```python
from build123d import *

# Parameters (mm, degrees)
SKETCH1_R           = 8
BOSS_EXTRUDE1_DEPTH = 40
CHAMFER1_SIZE       = 10
SKETCH2_R           = 8
BOSS_EXTRUDE2_DEPTH = 40
CUT_EXTRUDE2_REACH  = 134.076
SKETCH4_W           = 40
SKETCH4_H           = 10
FILLET4_R           = 10
CUT_EXTRUDE9_REACH  = 154.84
CUT_EXTRUDE10_REACH = 153.921
FILLET5_R           = 10
CUT_EXTRUDE11_REACH = 156.208
SKETCH15_R          = 12.5


with BuildPart() as part:
    # Sketch1 → Boss-Extrude1 (new body)
    with BuildSketch(Plane(origin=(0, 0, 0), x_dir=(1, 0, 0), z_dir=(0, 1, 0))):
        with BuildLine():
            Line((0, 0), (0, 144))
            Line((0, 144), (-6, 144))
            Line((-6, 144), (-6, 24))
            Line((-6, 24), (-26, 24))
            ThreePointArc((-26, 24), (-38, 12), (-26, 0))
            Line((-26, 0), (0, 0))
        make_face()
        with Locations(Location((-26, 12, 0), (0, 0, 270))):
            Circle(SKETCH1_R, mode=Mode.SUBTRACT)
    extrude(amount=BOSS_EXTRUDE1_DEPTH)

    # Chamfer1
    chamfer1_edges = [part.edges().sort_by_distance(p)[0] for p in [
        (-3, 40, -144),
        (-3, 0, -144),
    ]]
    chamfer(chamfer1_edges, length=CHAMFER1_SIZE)

    # Sketch2 → Boss-Extrude2 (add, through all)
    with BuildSketch(Plane(origin=(0, 40, 0), x_dir=(1, 0, 0), z_dir=(0, 1, 0))):
        with BuildLine():
            ThreePointArc((0, 0), (12, -12), (24, 0))
            Line((24, 0), (24, 24))
            Line((24, 24), (0, 24))
            Line((0, 24), (0, 0))
        make_face()
        with Locations(Location((12, 0, 0), (0, 0, 270))):
            Circle(SKETCH2_R, mode=Mode.SUBTRACT)
    extrude(amount=-BOSS_EXTRUDE2_DEPTH)

    # Sketch4 → Cut-Extrude2 (cut, up to next)
    with BuildSketch(Plane(origin=(0, 0, -24), x_dir=(-1, 0, 0), z_dir=(0, 0, -1)), mode=Mode.PRIVATE) as cut_extrude2_sk1:
        with Locations((26, 35)):
            Rectangle(SKETCH4_W, SKETCH4_H)
    cut_extrude2_tool1 = extrude(cut_extrude2_sk1.sketch, amount=-CUT_EXTRUDE2_REACH, mode=Mode.PRIVATE) & part.part
    # Sketch4 → Cut-Extrude2 (cut, up to next)
    with BuildSketch(Plane(origin=(0, 0, -24), x_dir=(-1, 0, 0), z_dir=(0, 0, -1)), mode=Mode.PRIVATE) as cut_extrude2_sk2:
        with Locations((26, 5)):
            Rectangle(SKETCH4_W, SKETCH4_H)
    cut_extrude2_tool2 = extrude(cut_extrude2_sk2.sketch, amount=-CUT_EXTRUDE2_REACH, mode=Mode.PRIVATE) & part.part
    # Sketch4 → Cut-Extrude2 (cut, up to next)
    with BuildSketch(Plane(origin=(0, 0, -24), x_dir=(-1, 0, 0), z_dir=(0, 0, -1)), mode=Mode.PRIVATE) as cut_extrude2_sk3:
        with Locations((-20, 5)):
            Rectangle(SKETCH4_W, SKETCH4_H)
    cut_extrude2_tool3 = extrude(cut_extrude2_sk3.sketch, amount=-CUT_EXTRUDE2_REACH, mode=Mode.PRIVATE) & part.part
    # Sketch4 → Cut-Extrude2 (cut, up to next)
    with BuildSketch(Plane(origin=(0, 0, -24), x_dir=(-1, 0, 0), z_dir=(0, 0, -1)), mode=Mode.PRIVATE) as cut_extrude2_sk4:
        with Locations((-20, 35)):
            Rectangle(SKETCH4_W, SKETCH4_H)
    cut_extrude2_tool4 = extrude(cut_extrude2_sk4.sketch, amount=-CUT_EXTRUDE2_REACH, mode=Mode.PRIVATE) & part.part
    add(cut_extrude2_tool1.solids().sort_by_distance((-26, 35, -24))[0], mode=Mode.SUBTRACT)
    add(cut_extrude2_tool2.solids().sort_by_distance((-26, 5, -24))[0], mode=Mode.SUBTRACT)
    add(cut_extrude2_tool3.solids().sort_by_distance((20, 5, -24))[0], mode=Mode.SUBTRACT)
    add(cut_extrude2_tool4.solids().sort_by_distance((20, 35, -24))[0], mode=Mode.SUBTRACT)

    # Fillet4
    fillet4_edges = [part.edges().sort_by_distance(p)[0] for p in [
        (-6, 20, -24),
    ]]
    fillet(fillet4_edges, radius=FILLET4_R)

    # Sketch13 → Cut-Extrude9 (cut, up to next)
    with BuildSketch(Plane.ZY.offset(6), mode=Mode.PRIVATE) as cut_extrude9_sk1:
        Polygon((0, 30), (-10, 40), (0, 40), align=None)
    cut_extrude9_tool1 = extrude(cut_extrude9_sk1.sketch, amount=-CUT_EXTRUDE9_REACH, mode=Mode.PRIVATE) & part.part
    # Sketch13 → Cut-Extrude9 (cut, up to next)
    with BuildSketch(Plane.ZY.offset(6), mode=Mode.PRIVATE) as cut_extrude9_sk2:
        Polygon((0, 10), (0, 0), (-10, 0), align=None)
    cut_extrude9_tool2 = extrude(cut_extrude9_sk2.sketch, amount=-CUT_EXTRUDE9_REACH, mode=Mode.PRIVATE) & part.part
    add(cut_extrude9_tool1.solids().sort_by_distance((-6, 36.666667, -3.333333))[0], mode=Mode.SUBTRACT)
    add(cut_extrude9_tool2.solids().sort_by_distance((-6, 3.333333, -3.333333))[0], mode=Mode.SUBTRACT)

    # Sketch14 → Cut-Extrude10 (cut, up to next)
    with BuildSketch(Plane(origin=(0, 30, 0), x_dir=(1, 0, 0), z_dir=(0, 1, 0)), mode=Mode.PRIVATE) as cut_extrude10_sk1:
        with BuildLine():
            Line((12, 12), (0, 12))
            Line((0, 12), (0, 24))
            Line((0, 24), (24, 24))
            Line((24, 24), (24, 0))
            ThreePointArc((24, 0), (20.485281374, 8.485281374), (12, 12))
        make_face()
    cut_extrude10_tool1 = extrude(cut_extrude10_sk1.sketch, amount=-CUT_EXTRUDE10_REACH, mode=Mode.PRIVATE) & part.part
    add(cut_extrude10_tool1.solids().sort_by_distance((12.903097, 30, -17.158841))[0], mode=Mode.SUBTRACT)

    # Fillet5
    # the kernel refuses this fillet: 10 mm, written as the material it adds along each edge
    with BuildSketch(Plane(origin=(0, 30, -12), x_dir=(0, 0, -1), z_dir=(0, -1, 0))) as fillet5_piece_1:
        with BuildLine():
            CenterArc((FILLET5_R, FILLET5_R), FILLET5_R, 180, 90)
            Line((0, FILLET5_R), (0, 0))
            Line((0, 0), (FILLET5_R, 0))
        make_face()
    extrude(amount=20)
    with BuildSketch(Plane(origin=(0, 10, 0), x_dir=(-1, 0, 0), z_dir=(0, 1, 0))) as fillet5_piece_2_section:
        with BuildLine():
            CenterArc((7.595917942, 10), FILLET5_R, 207.035691789, 62.964308211)
            ThreePointArc((-1.311317486, 5.454545455), (-0.332434055, 2.804978595), (0, 0))
            Line((0, 0), (7.595917942, 0))
        make_face()
    fillet5_piece_2 = extrude(amount=20, mode=Mode.PRIVATE)
    fillet5_piece_2 = split(fillet5_piece_2, bisect_by=Plane(origin=(-0.444204422, 11.816695322, 1.816695322), z_dir=(0, -0.7071067811865475, 0.7071067811865476)), keep=Keep.TOP, mode=Mode.PRIVATE)
    add(fillet5_piece_2)
    with BuildSketch(Plane(origin=(0, 10, 0), x_dir=(-1, 0, 0), z_dir=(0, 1, 0))) as fillet5_piece_3_section:
        with BuildLine():
            CenterArc((7.595917942, 10), FILLET5_R, 207.035691789, 62.964308211)
            ThreePointArc((-1.311317486, 5.454545455), (-0.332434055, 2.804978595), (0, 0))
            Line((0, 0), (7.595917942, 0))
        make_face()
    fillet5_piece_3 = extrude(amount=20, mode=Mode.PRIVATE)
    fillet5_piece_3 = split(fillet5_piece_3, bisect_by=Plane(origin=(-1.853866484, 24.485517863, 5.514482137), z_dir=(0, -0.7071067811865481, -0.707106781186547)), keep=Keep.TOP, mode=Mode.PRIVATE)
    fillet5_piece_3 = split(fillet5_piece_3, bisect_by=Plane(origin=(-1.853866484, 15.514482137, 5.514482137), z_dir=(0, 0.7071067811865475, -0.7071067811865476)), keep=Keep.TOP, mode=Mode.PRIVATE)
    add(fillet5_piece_3)
    with BuildSketch(Plane(origin=(0, 10, 0), x_dir=(-1, 0, 0), z_dir=(0, 1, 0))) as fillet5_piece_4_section:
        with BuildLine():
            CenterArc((7.595917942, 10), FILLET5_R, 207.035691789, 62.964308211)
            ThreePointArc((-1.311317486, 5.454545455), (-0.332434055, 2.804978595), (0, 0))
            Line((0, 0), (7.595917942, 0))
        make_face()
    fillet5_piece_4 = extrude(amount=20, mode=Mode.PRIVATE)
    fillet5_piece_4 = split(fillet5_piece_4, bisect_by=Plane(origin=(-0.444204422, 28.183304678, 1.816695322), z_dir=(0, 0.7071067811865481, 0.707106781186547)), keep=Keep.TOP, mode=Mode.PRIVATE)
    add(fillet5_piece_4)

    # Sketch15 → Cut-Extrude11 (cut, up to next)
    with BuildSketch(Plane(origin=(0, 0, 0), x_dir=(0, 0, -1), z_dir=(1, 0, 0)), mode=Mode.PRIVATE) as cut_extrude11_sk1:
        with Locations((83, 20)):
            Circle(SKETCH15_R)
    cut_extrude11_tool1 = extrude(cut_extrude11_sk1.sketch, amount=-CUT_EXTRUDE11_REACH, mode=Mode.PRIVATE) & part.part
    # Sketch15 → Cut-Extrude11 (cut, up to next)
    with BuildSketch(Plane(origin=(0, 0, 0), x_dir=(0, 0, -1), z_dir=(1, 0, 0)), mode=Mode.PRIVATE) as cut_extrude11_sk2:
        with Locations((118, 20)):
            Circle(SKETCH15_R)
    cut_extrude11_tool2 = extrude(cut_extrude11_sk2.sketch, amount=-CUT_EXTRUDE11_REACH, mode=Mode.PRIVATE) & part.part
    # Sketch15 → Cut-Extrude11 (cut, up to next)
    with BuildSketch(Plane(origin=(0, 0, 0), x_dir=(0, 0, -1), z_dir=(1, 0, 0)), mode=Mode.PRIVATE) as cut_extrude11_sk3:
        with Locations((48, 20)):
            Circle(SKETCH15_R)
    cut_extrude11_tool3 = extrude(cut_extrude11_sk3.sketch, amount=-CUT_EXTRUDE11_REACH, mode=Mode.PRIVATE) & part.part
    add(cut_extrude11_tool1.solids().sort_by_distance((0, 20, -83))[0], mode=Mode.SUBTRACT)
    add(cut_extrude11_tool2.solids().sort_by_distance((0, 20, -118))[0], mode=Mode.SUBTRACT)
    add(cut_extrude11_tool3.solids().sort_by_distance((0, 20, -48))[0], mode=Mode.SUBTRACT)


solid = part.part
```
CAD build for the part. Positions are in the model's coordinates, mm. Round coordinates to 2 decimals unless told otherwise and drop trailing zeros. Loops run counter-clockwise (first coordinate to the right, second up) from the corner with the lowest first, then second, coordinate; pieces in that order, holes last. Notation, with made-up numbers: M 85,34 L 117,34 A29 ccw 117,57 Z; hole C 67,62 d9. An arc over 180 degrees is marked long. Use a Markdown table: item, result. Add a question column.
(1) Drill centre lines: line 1 (Y direction, x = -2, z = -48); line 2 (Z direction, x = -3.5, y = 23); line 3 (Z direction, x = -26, y = 25). Where is each one in solid material? Low to high.
(2) Cut at B-B (z = -48). Give the cut face in (x, y).
(3) Cut at C-C (x = 13.5). Give the cut face in (y, z), and give its area (3 significant figures).
(4) Pull direction Z, two halves, no side cores. Call faces 1 (the face through (-3, 5, -5)), 2 (the face through (-9.01, 20.14, -26.85)), 3 (the face through (-33.81, 19.86, -13.73)): +Z half, -Z half, draft (parallel to the pull), parting line (faces both ways), or undercut.
(5) Flat gauge pins, fed straight in: pin 1 (9 mm diameter, centred on x = -17, y = 21, fed in from +Z); pin 2 (12 mm diameter, centred on y = 15, z = -53, fed in from +X); pin 3 (23 mm diameter, centred on x = -11.5, z = -19, fed in from -Y); pin 4 (5 mm diameter, centred on y = 29, z = -17, fed in from -X). Where does each tip first touch, or does it go through?
(6) Cut at D-D (y = 13.5). Give the cut face in (x, z).
(7) Cut at A-A (y = 20). Give the cut face in (x, z).
Geometry says:
| question | item | result |
|---|---|---|
| 1 | line 1 | y = 0 to 7.5, 32.5 to 40 |
| 1 | line 2 | z = -144 to -130.13, -105.87 to -95.13, -70.87 to -60.13, -35.87 to 0.88 |
| 1 | line 3 | z = -24 to -20, -4 to 0 |
| 2 | outline | M -6,0 L 0,0 L 0,7.5 L -6,7.5 Z; M -6,32.5 L 0,32.5 L 0,40 L -6,40 Z |
| 3 | outline | M 10,-11.91 L 30,-11.91 L 30,-7.86 L 10,-7.86 Z; M 10,7.86 L 30,7.86 L 30,11.91 L 10,11.91 Z |
| 3 | area | 162 mm² |
| 4 | face 1 | +Z half |
| 4 | face 2 | -Z half |
| 4 | face 3 | undercut |
| 5 | pin 1 | stops at z = 0 |
| 5 | pin 2 | stops at x = 0 |
| 5 | pin 3 | stops at y = 0 |
| 5 | pin 4 | stops at x = -37.74 |
| 6 | outline | M -26,-24 L -16,-24 A10 cw -6,-34 L -6,-37.32 L 0,-37.32 L 0,-22 A10 cw 10,-12 L 12,-12 A12 ccw long 1.31,5.45 A10 cw -7.6,0 L -26,0 A12 ccw Z; M -6,-144 L 0,-144 L 0,-128.68 L -6,-128.68 Z; M -6,-107.32 L 0,-107.32 L 0,-93.68 L -6,-93.68 Z; M -6,-72.32 L 0,-72.32 L 0,-58.68 L -6,-58.68 Z; hole C -26,-12 d16; hole C 12,0 d16 |
| 7 | outline | M -26,-24 L -16,-24 A10 cw -6,-34 L -6,-35.5 L 0,-35.5 L 0,-22 A10 cw 10,-12 L 12,-12 A12 ccw long 1.31,5.45 A10 cw -7.6,0 L -26,0 A12 ccw Z; M -6,-144 L 0,-144 L 0,-130.5 L -6,-130.5 Z; M -6,-105.5 L 0,-105.5 L 0,-95.5 L -6,-95.5 Z; M -6,-70.5 L 0,-70.5 L 0,-60.5 L -6,-60.5 Z; hole C -26,-12 d16; hole C 12,0 d16 |
